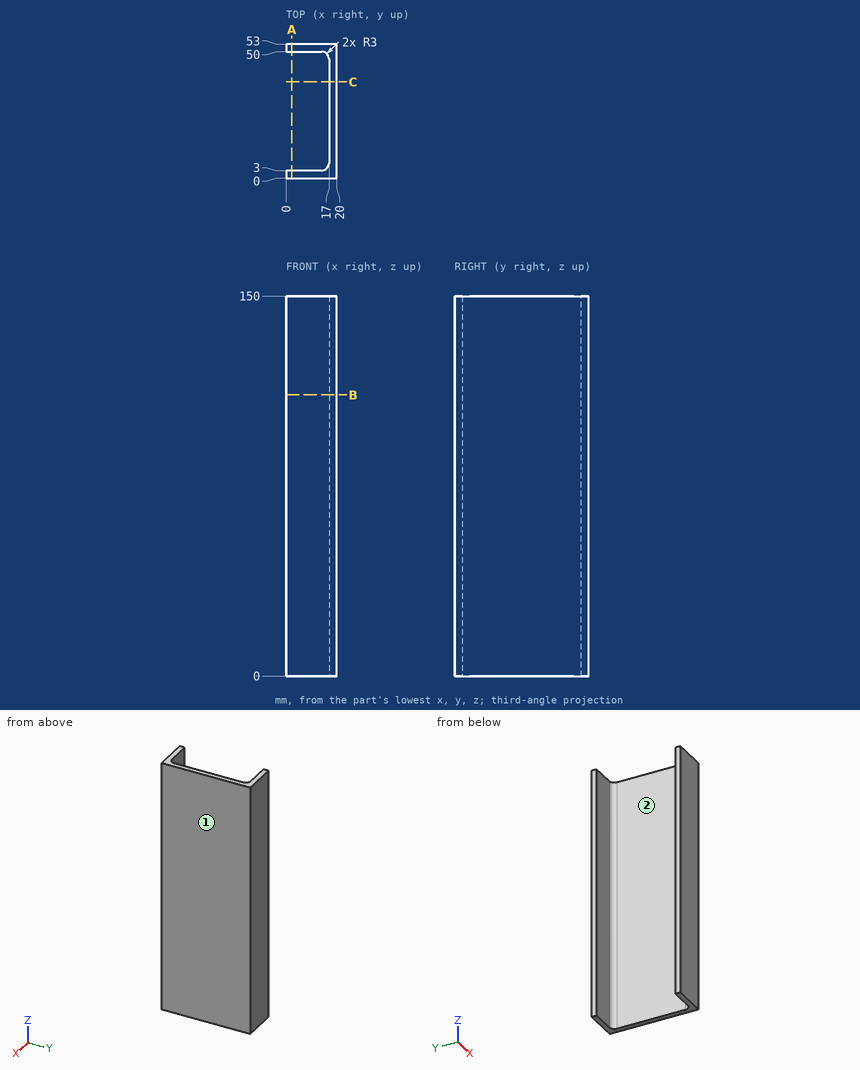
The drawing under review shows one solid part. Ordinate dimensions are in mm from its lowest x, y, z. A direction names the side the tool comes from. Coordinates: 2 decimals unless noted, no trailing zeros. Write each loop counter-clockwise with the first axis right and the second up, starting at its lowest first coordinate (ties: lowest second). Pieces come first, ordered by that corner, then holes. Notation, with made-up numbers: (87, 12) - (111, 12) arc R28 ccw to (111, 49) - close; hole circle Ø3 at (11, 25.5). An arc over 180 degrees is marked (long way). Put each result on its own line as item: value.
1. For pin 1 (3 mm diameter, centred on x = 7.5, z = 33, fed in from -Y); pin 2 (12.5 mm diameter, centred on y = 20.5, z = 97, fed in from -X); pin 3 (4 mm diameter, centred on x = 14, y = 47, fed in from +Z), all flat-tipped, find the tip position at first contact; note any pin that passes through.
Values found:
pin 1: y = 0
pin 2: x = 17
pin 3: through
2. Add section B-B, the plane z = 111. Give the boundary of the cut face in (x, y), then the cut area to 3 significant figures.
Values found:
outline: (0, 0) - (20, 0) - (20, 53) - (0, 53) - (0, 50) - (14, 50) arc R3 cw to (17, 47) - (17, 6) arc R3 cw to (14, 3) - (0, 3) - close
area: 265 mm²
3. Wall thickness on probe 1 along Y at (x, z) = (10.5, 66); probe 2 along X at (y, z) = (31.5, 109); probe 3 along Y at (x, z) = (16.25, 91): over which ranges is each line inside the solid? List them lowest first.
Values found:
probe 1: 0 to 3, 50 to 53
probe 2: 17 to 20
probe 3: 0 to 4.02, 48.98 to 53
4. Add section C-C, the plane y = 38. Give the boundary of the cut face in (x, z).
Values found:
outline: (17, 0) - (20, 0) - (20, 150) - (17, 150) - close
5. Machinability: for the marked faces 1 and 2, which of the approach directions +Z, -Z, +X, -X, +Y, -Y give a long, thin tool a straight path to every point of the face, cutting with its end or side? Answer none if there is none.
Values found:
face 1: +Z, -Z, +X, +Y, -Y
face 2: +Z, -Z, -X
6. Add section A-A, the plane x = 2.25. Give the boundary of the cut face in (y, z), then the cut area to 3 significant figures.
Values found:
outline: (0, 0) - (3, 0) - (3, 150) - (0, 150) - close; (50, 0) - (53, 0) - (53, 150) - (50, 150) - close
area: 900 mm²
